Input: part model. Units: mm. Frame: model coordinates. Face numbers are marked on the shaded views. A direction names the side the tool comes from. Coordinates: 2 decimals unless noted, no trailing zeros. Loops run counter-clockwise (first coordinate to the right, second up) from the corner with the lowest first, then second, coordinate; pieces in that order, holes last.
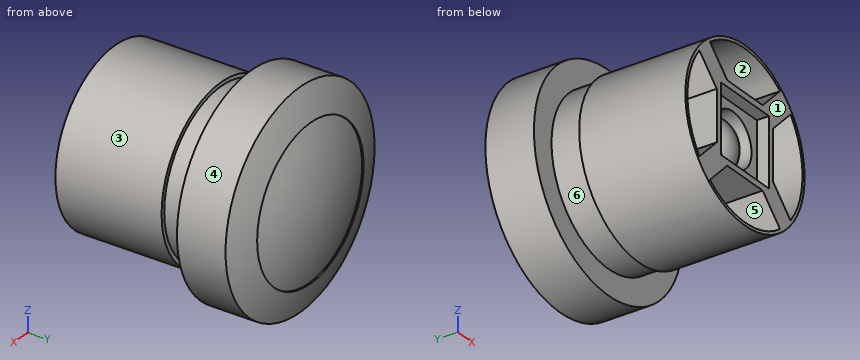
```python
from build123d import *

# Parameters (mm, degrees)
SKETCH1_R           = 5.6
BOSS_EXTRUDE1_DEPTH = 9
SKETCH4_R           = 5.6
SKETCH4_R_2         = 5.35
CUT_EXTRUDE1_DEPTH  = 2
SKETCH5_R           = 5.4
CUT_EXTRUDE3_DEPTH  = 6
BOSS_EXTRUDE2_DEPTH = 6
SKETCH7_W           = 4.5
SKETCH7_H           = 4.5
CUT_EXTRUDE4_DEPTH  = 0.8
SKETCH8_R           = 1.75
CUT_EXTRUDE5_DEPTH  = 1


with BuildPart() as part:
    # Sketch1 → Boss-Extrude1 (new body)
    with BuildSketch(Plane(origin=(0, 0, 0), x_dir=(1, 0, 0), z_dir=(0, 1, 0))):
        Circle(SKETCH1_R)
    extrude(amount=BOSS_EXTRUDE1_DEPTH)

    # Sketch2 → Revolve1 (revolve)
    with BuildSketch(Plane.XY):
        with BuildLine():
            Line((0, 9), (0, 13.7))
            ThreePointArc((0, 13.7), (-2.541861151, 13.468387517), (-5, 12.78117878))
            Line((-5, 12.78117878), (-5, 12.88117878))
            ThreePointArc((-5, 12.88117878), (-6.008472362, 12.565464979), (-7, 12.2))
            Line((-7, 12.2), (-7, 9))
            Line((-7, 9), (0, 9))
        make_face()
    revolve(axis=Axis((0, 9, 0), (0, 1, 0)))

    # Sketch4 → Cut-Extrude1 (cut)
    with BuildSketch(Plane.XZ.offset(-9)):
        Circle(SKETCH4_R)
        Circle(SKETCH4_R_2, mode=Mode.SUBTRACT)
    extrude(amount=CUT_EXTRUDE1_DEPTH, mode=Mode.SUBTRACT)

    # Sketch5 → Cut-Extrude3 (cut)
    with BuildSketch(Plane.XZ):
        Circle(SKETCH5_R)
    extrude(amount=-CUT_EXTRUDE3_DEPTH, mode=Mode.SUBTRACT)

    # Sketch6 → Boss-Extrude2 (add)
    with BuildSketch(Plane.XZ):
        with BuildLine():
            Line((3.291184257, -4.28113375), (1.660050506, -2.65))
            Line((1.660050506, -2.65), (-1.660050506, -2.65))
            Line((-1.660050506, -2.65), (-3.291184257, -4.28113375))
            ThreePointArc((-3.291184257, -4.28113375), (-3.818376618, -3.818376618), (-4.28113375, -3.291184257))
            Line((-4.28113375, -3.291184257), (-2.65, -1.660050506))
            Line((-2.65, -1.660050506), (-2.65, 1.660050506))
            Line((-2.65, 1.660050506), (-4.28113375, 3.291184257))
            ThreePointArc((-4.28113375, 3.291184257), (-3.818376618, 3.818376618), (-3.291184257, 4.28113375))
            Line((-3.291184257, 4.28113375), (-1.660050506, 2.65))
            Line((-1.660050506, 2.65), (1.660050506, 2.65))
            Line((1.660050506, 2.65), (3.291184257, 4.28113375))
            ThreePointArc((3.291184257, 4.28113375), (3.818376618, 3.818376618), (4.28113375, 3.291184257))
            Line((4.28113375, 3.291184257), (2.65, 1.660050506))
            Line((2.65, 1.660050506), (2.65, -1.660050506))
            Line((2.65, -1.660050506), (4.28113375, -3.291184257))
            ThreePointArc((4.28113375, -3.291184257), (3.818376618, -3.818376618), (3.291184257, -4.28113375))
        make_face()
    extrude(amount=-BOSS_EXTRUDE2_DEPTH)

    # Sketch7 → Cut-Extrude4 (cut)
    with BuildSketch(Plane.XZ):
        Rectangle(SKETCH7_W, SKETCH7_H)
    extrude(amount=-CUT_EXTRUDE4_DEPTH, mode=Mode.SUBTRACT)

    # Sketch8 → Cut-Extrude5 (cut)
    with BuildSketch(Plane.XZ.offset(-0.8)):
        Circle(SKETCH8_R)
    extrude(amount=-CUT_EXTRUDE5_DEPTH, mode=Mode.SUBTRACT)

    # Sketch9 → Revolve2 (revolve)
    with BuildSketch(Plane.XY):
        with BuildLine():
            Line((0, 0.8), (0, 1.8))
            Line((0, 1.8), (-1.75, 1.8))
            ThreePointArc((-1.75, 1.8), (-1.007782219, 1.067631118), (0, 0.8))
        make_face()
    revolve(axis=Axis((0, 0.8, 0), (0, 1, 0)))


solid = part.part
```
Item 1: Section query B-B (y = 10.25). Output: boundary loops of the cut face in (x, z), then the cut area to 3 significant figures.
Result:
outline: circle Ø14 at (0, 0)
area: 154 mm2
Item 2: Section query C-C (y = 7.75). Output: boundary loops of the cut face in (x, z).
Result:
outline: circle Ø10.7 at (0, 0)
Item 3: Contact query for flat-ended pins moving along their axis: P1, Ø1.5, axis at x = -3.5, y = 3, coming from the -Z side; P2, Ø3, axis at x = -0.5, z = 4, coming from the -Y side; P3, Ø5, axis at x = 4.5, y = 12, coming from the +Z side; P4, Ø2.5, axis at x = 0, y = 2.5, coming from the -Z side. Output: stop coordinate, or through.
Result:
P1: stops at z = -4.88
P2: stops at y = 0
P3: stops at z = 6.71
P4: stops at z = -5.6
Item 4: Line query: L1, parallel to Z at x = -1.75, y = 2; L2, parallel to Z at x = -1, y = 5.5. Output: solid intervals per line, ascending.
Result:
L1: z = -5.32 to -5.11, -2.74 to 2.74, 5.11 to 5.32
L2: z = -5.51 to -5.31, -2.65 to 2.65, 5.31 to 5.51
Item 5: Reachability of the marked faces 4, 5 and 6 from +Z, -Z, +X, -X, +Y, -Y: full face, straight path, thin tool, end or side. Return the list, or none.
Result:
face 4: +Y, -Y
face 5: -Y
face 6: none
Item 6: Section query A-A (y = 4.5). Output: boundary loops of the cut face in (x, z), then the cut area to 3 significant figures.
Result:
outline: circle Ø11.2 at (0, 0); hole (-4.28, -3.29) - (-2.65, -1.66) - (-2.65, 1.66) - (-4.28, 3.29) arc R5.4 ccw to start; hole (-3.29, -4.28) arc R5.4 ccw to (3.29, -4.28) - (1.66, -2.65) - (-1.66, -2.65) - close; hole (-3.29, 4.28) - (-1.66, 2.65) - (1.66, 2.65) - (3.29, 4.28) arc R5.4 ccw to start; hole (2.65, -1.66) - (4.28, -3.29) arc R5.4 ccw to (4.28, 3.29) - (2.65, 1.66) - close
area: 46.1 mm2
Item 7: Mould query, pull axis Z, two halves, no side actions, for the marked faces 1, 2 and 3. Classes: +Z half, -Z half, draft (parallel to the pull), parting line (faces both ways), or undercut.
Result:
face 1: draft
face 2: undercut
face 3: parting line
